from build123d import *

# Parameters (mm, degrees)
BOSS_EXTRUDE1_DEPTH = 20
CUT_EXTRUDE23_DEPTH = 444
CUT_EXTRUDE26_DEPTH = 444
BOSS_EXTRUDE2_DEPTH = 14
SKETCH15_R          = 2.72
CUT_EXTRUDE27_DEPTH = 14
SKETCH16_R          = 3.25
SKETCH16_R_2        = 3.15
CUT_EXTRUDE28_DEPTH = 45
CUT_EXTRUDE29_DEPTH = 6.15
CUT_EXTRUDE31_DEPTH = 45
SKETCH18_R          = 3.2
CUT_EXTRUDE32_DEPTH = 45


with BuildPart() as part:
    # Sketch1 → Boss-Extrude1 (new body)
    with BuildSketch(Plane(origin=(0, 0, 0), x_dir=(1, 0, 0), z_dir=(0, 1, 0))):
        Polygon((-22.5, 328), (-17.5, 328), (-17.5, 352.208543952), (-12.5, 352.208543952), (-12.5, 328), (-7.5, 328), (-7.5, 352.208543952), (-2.5, 352.208543952), (2.5, 352.208543952), (7.5, 352.208543952), (7.5, 328), (12.5, 328), (12.5, 352.208543952), (17.5, 352.208543952), (17.5, 328), (22.5, 328), (22.5, 392.208543952), (-22.5, 392.208543952), align=None)
    extrude(amount=BOSS_EXTRUDE1_DEPTH)

    # Sketch2 → Cut-Extrude23 (cut)
    with BuildSketch(Plane.XY.offset(50)):
        with BuildLine():
            Line((-22.5, 20), (22.5, 20))
            Line((22.5, 20), (22.5, 16))
            ThreePointArc((22.5, 16), (20.832845478, 17.631987193), (18.5, 17.607120136))
            ThreePointArc((18.5, 17.607120136), (0, 13.071891388), (-18.5, 17.607120136))
            ThreePointArc((-18.5, 17.607120136), (-20.832845478, 17.631987193), (-22.5, 16))
            Line((-22.5, 16), (-22.5, 20))
        make_face()
    extrude(amount=-CUT_EXTRUDE23_DEPTH, mode=Mode.SUBTRACT)

    # Sketch12 → Cut-Extrude26 (cut)
    with BuildSketch(Plane.XY.offset(50)):
        Polygon((-1, 3.35), (-1, 6.55), (0, 6.55), (1, 6.55), (1, 3.35), align=None)
    extrude(amount=-CUT_EXTRUDE26_DEPTH, mode=Mode.SUBTRACT)

    # Sketch14 → Boss-Extrude2 (add)
    with BuildSketch(Plane(origin=(0, 0, -392.208543952), x_dir=(-1, 0, 0), z_dir=(0, 0, -1))):
        with BuildLine():
            Line((-22.5, 0), (-22.5, -20))
            ThreePointArc((-22.5, -20), (0, -42.5), (22.5, -20))
            Line((22.5, -20), (22.5, 0))
            Line((22.5, 0), (-22.5, 0))
        make_face()
    extrude(amount=-BOSS_EXTRUDE2_DEPTH)

    # Sketch15 → Cut-Extrude27 (cut)
    with BuildSketch(Plane(origin=(0, 0, -392.208543952), x_dir=(-1, 0, 0), z_dir=(0, 0, -1))):
        with Locations((11.25, -20)):
            Circle(SKETCH15_R)
        with Locations((0, -6.75)):
            Circle(SKETCH15_R)
        with Locations((-11.25, -20)):
            Circle(SKETCH15_R)
        with Locations((0, -31.25)):
            Circle(SKETCH15_R)
    extrude(amount=-CUT_EXTRUDE27_DEPTH, mode=Mode.SUBTRACT)

    # Sketch16 → Cut-Extrude28 (cut)
    with BuildSketch(Plane.ZY.offset(22.5)):
        with Locations((-1.25, 8.5)):
            Circle(SKETCH16_R)
        with Locations((-386.058543952, 2.588831384)):
            Circle(SKETCH16_R_2)
    extrude(amount=-CUT_EXTRUDE28_DEPTH, mode=Mode.SUBTRACT)

    # Sketch17 → Cut-Extrude29 (cut)
    with BuildSketch(Plane(origin=(0, 0, -392.208543952), x_dir=(-1, 0, 0), z_dir=(0, 0, -1))):
        Polygon((1, 8.5), (5, 8.5), (5, 2.5), (-5, 2.5), (-5, 8.5), (-1, 8.5), align=None)
    extrude(amount=-CUT_EXTRUDE29_DEPTH, mode=Mode.SUBTRACT)

    # Sketch8 → Cut-Extrude31 (cut)
    with BuildSketch(Plane(origin=(22.5, 0, 0), x_dir=(0, 0, -1), z_dir=(1, 0, 0))):
        with BuildLine():
            ThreePointArc((336.5, 0), (330.48959236, 2.48959236), (328, 8.5))
            Line((328, 8.5), (328, 0))
            Line((328, 0), (336.5, 0))
        make_face()
        with BuildLine():
            Line((336.5, 20), (328, 20))
            Line((328, 20), (328, 17))
            Line((328, 17), (328, 8.5))
            ThreePointArc((328, 8.5), (330.48959236, 14.51040764), (336.5, 17))
            Line((336.5, 17), (348, 17))
            Line((348, 17), (348, 20))
            Line((348, 20), (336.5, 20))
        make_face()
    extrude(amount=-CUT_EXTRUDE31_DEPTH, mode=Mode.SUBTRACT)

    # Sketch18 → Cut-Extrude32 (cut)
    with BuildSketch(Plane(origin=(22.5, 0, 0), x_dir=(0, 0, -1), z_dir=(1, 0, 0))):
        with Locations((338, 8.5)):
            Circle(SKETCH18_R)
    extrude(amount=-CUT_EXTRUDE32_DEPTH, mode=Mode.SUBTRACT)


solid = part.part
CAD build for the part. Positions are in the model's coordinates, mm. A direction names the side the tool comes from. Coordinates: 2 decimals unless noted, no trailing zeros. Order: outer loops, then holes, each group sorted by start corner. A loop starts at its lowest first (then second) coordinate and runs counter-clockwise, first axis right, second up. Notation, with made-up numbers: (43.25, 73.25) -> (90.25, 73.25) arc R13 cw to (90.25, 77.25) -> close; hole circle Ø2 at (31, 54.25). An arc over 180 degrees is marked (long way). Answer in a Markdown table with one row per item.
1) Band-saw the part on B-B (z = -338). Give the number of separate pieces and of enclosed holes in the cut face, and give its area (3 significant figures).
Check values:
| item | result |
|---|---|
| separate pieces | 8 |
| enclosed holes | 0 |
| area | 185 mm2 |
2) Band-saw the part on D-D (y = -31.25). List the corners of the cut face in (x, z).
Check values:
| item | result |
|---|---|
| outline | (-19.49, -392.21) -> (-2.72, -392.21) -> (-2.72, -378.21) -> (-19.49, -378.21) -> close; (2.72, -392.21) -> (19.49, -392.21) -> (19.49, -378.21) -> (2.72, -378.21) -> close |
3) Drill centre lines: line 1 (Y direction, x = 11, z = -386); line 2 (Z direction, x = -15.5, y = 9); line 3 (Z direction, x = -14.5, y = 2.5). Where is each one in solid material? Low to high.
Check values:
| item | result |
|---|---|
| line 1 | -39.63 to -22.71, -17.29 to -0.56, 5.74 to 14.61 |
| line 2 | -392.21 to -352.21 |
| line 3 | -392.21 to -389.21, -382.91 to -352.21 |
4) Band-saw the part on C-C (x = 0). List the corners of the cut face in (y, z).
Check values:
| item | result |
|---|---|
| outline | (-42.5, -392.21) -> (-33.97, -392.21) -> (-33.97, -378.21) -> (-42.5, -378.21) -> close; (-28.53, -392.21) -> (-9.47, -392.21) -> (-9.47, -378.21) -> (-28.53, -378.21) -> close; (-4.03, -392.21) -> (2.5, -392.21) -> (2.5, -389.21) arc R3.15 cw (long way) to (3.35, -383) -> (3.35, -352.21) -> (0, -352.21) -> (0, -378.21) -> (-4.03, -378.21) -> close; (6.55, -386.06) -> (8.5, -386.06) -> (8.5, -392.21) -> (13.07, -392.21) -> (13.07, -352.21) -> (6.55, -352.21) -> close |
5) Mould opens along X. For faces 6 (the face through (0, -21, -378.209)), 7 (the face through (22.5, 2, -368)), 8 (the face through (-17.5, 8, -343)), 9 (the face through (0, 2.5, -391)) say: pulls with the +X half, pulls with the -X half, needs draft (parallel to the pull), parting line crosses it, or undercut.
Check values:
| item | result |
|---|---|
| face 6 | needs draft |
| face 7 | pulls with the +X half |
| face 8 | undercut |
| face 9 | undercut |
6) Which spindle directions (+Z, -Z, +X, -X, +Y, -Y) get a long thin tool onto all of the face, cutting with end or side? Do faces 1 (the face through (-9.965, 7.274, -340.956)), 2 (the face through (-1, 5, -369)), 3 (the face through (-20, 17, -342)), 4 (the face through (0, 7, -352.209)), 5 (the face through (0, 0, -362)). Say none if no direction does.
Check values:
| item | result |
|---|---|
| face 1 | +X, -X |
| face 2 | +Z, -Z |
| face 3 | +Z, +X, -X, +Y |
| face 4 | +Z, +Y, -Y |
| face 5 | +Z, +X, -X, -Y |
7) Band-saw the part on A-A (y = -6.75). List the corners of the cut face in (x, z).
Check values:
| item | result |
|---|---|
| outline | (-22.5, -392.21) -> (-2.72, -392.21) -> (-2.72, -378.21) -> (-22.5, -378.21) -> close; (2.72, -392.21) -> (22.5, -392.21) -> (22.5, -378.21) -> (2.72, -378.21) -> close |
8) Flat gauge pins, fed straight in: P1, Ø6.5, axis at x = -11.25, y = -20, coming from the +Z side; P2, Ø1.3, axis at x = -19.5, z = -343.5, coming from the +Y side; P3, Ø0.9, axis at x = -18.5, y = 17.5, coming from the +Z side. Where does each tip first touch, or does it go through?
Check values:
| item | result |
|---|---|
| P1 | z = -378.21 |
| P2 | y = 17 |
| P3 | z = -348 |
